from build123d import *

# Parameters (mm, degrees)
BOSS_EXTRU_1_DEPTH      = 3
ENL_V_MAT_EXTRU_1_DEPTH = 395.818945847
ESQUISSE3_R             = 1.6
ENL_V_MAT_EXTRU_2_DEPTH = 395.818945847


with BuildPart() as part:
    # Esquisse1 → Boss.-Extru.1 (new body)
    with BuildSketch(Plane.XY):
        with BuildLine():
            Line((7, 0), (240, 0))
            ThreePointArc((240, 0), (244.949747468, 2.050252532), (247, 7))
            Line((247, 7), (247, 301))
            ThreePointArc((247, 301), (244.949747468, 305.949747468), (240, 308))
            Line((240, 308), (7, 308))
            ThreePointArc((7, 308), (2.050252532, 305.949747468), (0, 301))
            Line((0, 301), (0, 7))
            ThreePointArc((0, 7), (2.050252532, 2.050252532), (7, 0))
        make_face()
    extrude(amount=BOSS_EXTRU_1_DEPTH)

    # Esquisse2 → Enlèv. mat.-Extru.1 (cut, through all)
    with BuildSketch(Plane(origin=(0, 0, 0), x_dir=(-1, 0, 0), z_dir=(0, 0, -1))):
        with BuildLine():
            Line((-54, 289.5), (-67, 289.5))
            Line((-67, 289.5), (-67, 281.5))
            ThreePointArc((-67, 281.5), (-60.5, 275), (-54, 281.5))
            Line((-54, 281.5), (-54, 289.5))
        make_face()
        with BuildLine():
            Line((-193, 289.5), (-193, 281.5))
            ThreePointArc((-193, 281.5), (-186.5, 275), (-180, 281.5))
            Line((-180, 281.5), (-180, 289.5))
            Line((-180, 289.5), (-180, 289.526253408))
            Line((-180, 289.526253408), (-193, 289.526253408))
            Line((-193, 289.526253408), (-193, 289.5))
        make_face()
    extrude(amount=-ENL_V_MAT_EXTRU_1_DEPTH, mode=Mode.SUBTRACT)

    # Esquisse3 → Enlèv. mat.-Extru.2 (cut, through all)
    with BuildSketch(Plane(origin=(0, 0, 0), x_dir=(-1, 0, 0), z_dir=(0, 0, -1))):
        with Locations((-170.55, 88.75)):
            Circle(ESQUISSE3_R)
        with Locations(Location((-76.45, 40.21, 0), (0, 0, 180))):
            Circle(ESQUISSE3_R)
        with Locations((-170.55, 40.21)):
            Circle(ESQUISSE3_R)
        with Locations(Location((-76.45, 88.75, 0), (0, 0, 180))):
            Circle(ESQUISSE3_R)
        with BuildLine():
            Line((-158.22, 88.96), (-88.78, 88.96))
            ThreePointArc((-88.78, 88.96), (-87.365786438, 88.374213562), (-86.78, 86.96))
            Line((-86.78, 86.96), (-86.78, 42))
            ThreePointArc((-86.78, 42), (-87.365786438, 40.585786438), (-88.78, 40))
            Line((-88.78, 40), (-158.22, 40))
            ThreePointArc((-158.22, 40), (-159.634213562, 40.585786438), (-160.22, 42))
            Line((-160.22, 42), (-160.22, 86.96))
            ThreePointArc((-160.22, 86.96), (-159.634213562, 88.374213562), (-158.22, 88.96))
        make_face()
    extrude(amount=-ENL_V_MAT_EXTRU_2_DEPTH, mode=Mode.SUBTRACT)


solid = part.part
The listing builds one solid part. Answer for the finished solid, in the listing's coordinates (mm). A direction names the side the tool comes from. Give positions to 0.01 mm unless a question says otherwise; leave off trailing zeros. Write each loop counter-clockwise with the first axis right and the second up, starting at its lowest first coordinate (ties: lowest second). Pieces come first, ordered by that corner, then holes.
1) Section B-B (y = 54) is taken. Write down the section's boundary in (x, z).
2) A tool of negligible diameter and unlimited length cuts with its end or side. For faces 1 (the face through (60.6, 275, 1.5)), 2 (the face through (2, 2.1, 1.5)), from which of +Z, -Z, +X, -X, +Y, -Y can it reach the whole face along a straight path? Write none if from no direction.
3) For a pull along X with two mould halves and no side action, classify faces 3 (the face through (186.6, 275, 1.5)), 4 (the face through (122, 156, 3)), 5 (the face through (2.1, 306, 1.5)), 6 (the face through (245, 305.9, 1.5)) as pulls with the +X half, pulls with the -X half, needs draft (parallel to the pull), parting line crosses it, or undercut.
4) Section A-A (z = 1.75) is taken. Write down the section's boundary in (x, y), and give its area (3 significant figures).
5) Given P1, Ø4, axis at x = 170.55, y = 40.21, coming from the +Z side; P2, Ø1.9, axis at x = 76.45, y = 40.21, coming from the +Z side, each flat-ended and moving along its own axis, determine where each tip first touches the part or whether it passes through.
6) Section C-C (x = 186.5) is taken. Write down the section's boundary in (y, z).
7) Find the intervals of material crossed by L1, parallel to Y at x = 76.45, z = 1.5; L2, parallel to X at y = 288, z = 2.4; L3, parallel to Y at x = 113.5, z = 0.4, in increasing order.
Response:
1. outline: (0, 0) - (86.78, 0) - (86.78, 3) - (0, 3) - close; (160.22, 0) - (247, 0) - (247, 3) - (160.22, 3) - close
2. face 1: +Z, -Z
2. face 2: +Z, -Z, -X, -Y
3. face 3: undercut
3. face 4: needs draft
3. face 5: pulls with the -X half
3. face 6: pulls with the +X half
4. outline: (0, 7) arc R7 ccw to (7, 0) - (240, 0) arc R7 ccw to (247, 7) - (247, 301) arc R7 ccw to (240, 308) - (7, 308) arc R7 ccw to (0, 301) - close; hole (54, 281.5) arc R6.5 ccw to (67, 281.5) - (67, 289.5) - (54, 289.5) - close; hole circle Ø3.2 at (76.45, 40.21); hole circle Ø3.2 at (76.45, 88.75); hole (86.78, 42) arc R2 ccw to (88.78, 40) - (158.22, 40) arc R2 ccw to (160.22, 42) - (160.22, 86.96) arc R2 ccw to (158.22, 88.96) - (88.78, 88.96) arc R2 ccw to (86.78, 86.96) - close; hole circle Ø3.2 at (170.55, 40.21); hole circle Ø3.2 at (170.55, 88.75); hole (180, 281.5) arc R6.5 ccw to (193, 281.5) - (193, 289.53) - (180, 289.53) - close
4. area: 72,100 mm2
5. P1: stops at z = 3
5. P2: passes through
6. outline: (0, 0) - (275, 0) - (275, 3) - (0, 3) - close; (289.53, 0) - (308, 0) - (308, 3) - (289.53, 3) - close
7. L1: y = 0 to 38.61, 41.81 to 87.15, 90.35 to 308
7. L2: x = 0 to 54, 67 to 180, 193 to 247
7. L3: y = 0 to 40, 88.96 to 308
